Source: CAD feature listing. Evaluate the final solid. Frame: model axes, mm. Face numbers are marked on the shaded views. A direction names the side the tool comes from. Round coordinates to 2 decimals unless told otherwise and drop trailing zeros. Order: outer loops, then holes, each group sorted by start corner. A loop starts at its lowest first (then second) coordinate and runs counter-clockwise, first axis right, second up. Notation, with made-up numbers: (-21, 54) - (19, 54) arc R21 cw to (19, 69) - close; hole circle Ø7 at (15.25, -9.5). An arc over 180 degrees is marked (long way). Return JSON: item names as keys, results as strings. Group by question number.
1) Access query for the marked faces 4 and 5. Directions: +Z, -Z, +X, -X, +Y, -Y. A direction counts if a zero-diameter tool reaches every point of the face in a straight line with its end or side. Return the directions, or none.
2) Section A-A, the plane x = 40.5. Return loops of the section in (y, z).
3) Mould query, pull axis X, two halves, no side actions, for the marked faces 1, 2 and 3. Classes: pulls with the +X half, pulls with the -X half, needs draft (parallel to the pull), parting line crosses it, or undercut.
4) Section D-D, the plane y = -76.5. Return loops of the section in (x, z), plus the area to 3 significant figures.
5) Section B-B, the plane z = 55. Return loops of the section in (x, y), plus the area to 3 significant figures.
6) Contact query for flat-ended pins moving along their axis: P1, Ø1.8, axis at y = -210, z = 65, coming from the +X side; P2, Ø12, axis at x = 167, z = 15, coming from the -Y side; P3, Ø2, axis at x = 236.5, z = 22, coming from the -Y side; P4, Ø1.8, axis at y = -210, z = 56.5, coming from the -X side. Output: stop coordinate, or through.
7) Section C-C, the plane z = 24. Return loops of the section in (x, y), plus the area to 3 significant figures.
8) Ray query, line 1 (X direction, y = -23.5, z = 40); line 2 (Y direction, x = -29, z = 85); line 3 (Z direction, x = 179.5, y = -192.5). Return the intervals inside material, ascending. Write a range as from..to.
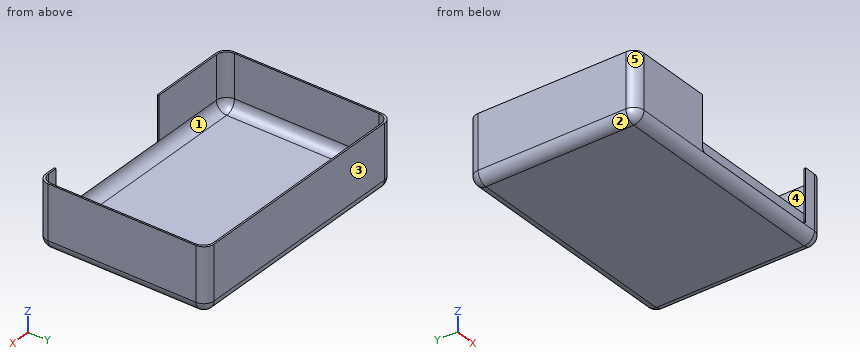
```python
from build123d import *

# Parameters (mm, degrees)
BOSS_EXTRUDE1_DEPTH = 88.9
CUT_EXTRUDE1_DEPTH  = 73.914
FILLET1_R           = 14.224
FILLET2_R           = 14.224
CUT_EXTRUDE2_DEPTH  = 2.286


with BuildPart() as part:
    # Sketch1 → Boss-Extrude1 (new body)
    with BuildSketch(Plane.XY):
        with BuildLine():
            Line((-41.405944168, 22.056216238), (266.696055832, 22.056216238))
            ThreePointArc((266.696055832, 22.056216238), (276.753942688, 17.890103094), (280.920055832, 7.832216238))
            Line((280.920055832, 7.832216238), (280.920055832, -197.145783762))
            ThreePointArc((280.920055832, -197.145783762), (276.753942688, -207.203670617), (266.696055832, -211.369783762))
            Line((266.696055832, -211.369783762), (-41.405944168, -211.369783762))
            ThreePointArc((-41.405944168, -211.369783762), (-51.463831024, -207.203670617), (-55.629944168, -197.145783762))
            Line((-55.629944168, -197.145783762), (-55.629944168, 7.832216238))
            ThreePointArc((-55.629944168, 7.832216238), (-51.463831024, 17.890103094), (-41.405944168, 22.056216238))
        make_face()
    extrude(amount=BOSS_EXTRUDE1_DEPTH)

    # Sketch4 → Cut-Extrude1 (cut)
    with BuildSketch(Plane.XY.offset(88.9)):
        with BuildLine():
            Line((-39.119944168, -209.083783762), (264.410055832, -209.083783762))
            ThreePointArc((264.410055832, -209.083783762), (274.467942688, -204.917670617), (278.634055832, -194.859783762))
            Line((278.634055832, -194.859783762), (278.634055832, 5.546216238))
            ThreePointArc((278.634055832, 5.546216238), (274.467942688, 15.604103094), (264.410055832, 19.770216238))
            Line((264.410055832, 19.770216238), (-39.119944168, 19.770216238))
            ThreePointArc((-39.119944168, 19.770216238), (-49.177831024, 15.604103094), (-53.343944168, 5.546216238))
            Line((-53.343944168, 5.546216238), (-53.343944168, -194.859783762))
            ThreePointArc((-53.343944168, -194.859783762), (-49.177831024, -204.917670617), (-39.119944168, -209.083783762))
        make_face()
    extrude(amount=-CUT_EXTRUDE1_DEPTH, mode=Mode.SUBTRACT)

    # Fillet1
    fillet1_edges = [part.edges().sort_by_distance(p)[0] for p in [
        (-49.177831024, -204.917670617, 14.986),
        (-53.343944168, -94.656783762, 14.986),
        (-49.177831024, 15.604103094, 14.986),
        (112.645055832, 19.770216238, 14.986),
        (274.467942688, 15.604103094, 14.986),
        (278.634055832, -94.656783762, 14.986),
        (274.467942688, -204.917670617, 14.986),
        (112.645055832, -209.083783762, 14.986),
    ]]
    fillet(fillet1_edges, radius=FILLET1_R)

    # Fillet2
    fillet2_edges = [part.edges().sort_by_distance(p)[0] for p in [
        (-55.629944168, -94.656783762, 0),
        (-51.463831024, 17.890103094, 0),
        (112.645055832, 22.056216238, 0),
        (276.753942688, 17.890103094, 0),
        (280.920055832, -94.656783762, 0),
        (276.753942688, -207.203670617, 0),
        (112.645055832, -211.369783762, 0),
        (-51.463831024, -207.203670617, 0),
    ]]
    fillet(fillet2_edges, radius=FILLET2_R)

    # Sketch5 → Cut-Extrude2 (cut)
    with BuildSketch(Plane(origin=(0, -211.369783762, 0), x_dir=(-1, 0, 0), z_dir=(0, -1, 0))):
        with BuildLine():
            Line((-69.838151491, -14.224), (-245.885767903, -14.224))
            ThreePointArc((-245.885767903, -14.224), (-249.477870351, -15.711897552), (-250.965767903, -19.304))
            Line((-250.965767903, -19.304), (-250.965767903, -88.9))
            Line((-250.965767903, -88.9), (-64.758151491, -88.9))
            Line((-64.758151491, -88.9), (-64.758151491, -19.304))
            ThreePointArc((-64.758151491, -19.304), (-66.246049042, -15.711897552), (-69.838151491, -14.224))
        make_face()
    extrude(amount=-CUT_EXTRUDE2_DEPTH, mode=Mode.SUBTRACT)


solid = part.part
```
Geometry check:
{
 "1": {"face 4": "+Z", "face 5": "+Z, -Z, -X, -Y"},
 "2": {"outline": "(-211.37, 14.22) arc R14.22 ccw to (-197.15, 0) - (7.83, 0) arc R14.22 ccw to (22.06, 14.22) - (22.06, 88.9) - (19.77, 88.9) - (19.77, 29.21) arc R14.22 cw to (5.55, 14.99) - (-194.86, 14.99) arc R14.22 cw to (-209.08, 29.21) - (-209.08, 88.9) - (-211.37, 88.9) - close"},
 "3": {"face 1": "undercut", "face 2": "pulls with the -X half", "face 3": "needs draft"},
 "4": {"outline": "(-55.63, 14.22) arc R14.22 ccw to (-41.41, 0) - (266.7, 0) arc R14.22 ccw to (280.92, 14.22) - (280.92, 88.9) - (278.63, 88.9) - (278.63, 29.21) arc R14.22 cw to (264.41, 14.99) - (-39.12, 14.99) arc R14.22 cw to (-53.34, 29.21) - (-53.34, 88.9) - (-55.63, 88.9) - close", "area": "5,380 mm2"},
 "5": {"outline": "(-55.63, -197.15) arc R14.22 ccw to (-41.41, -211.37) - (64.76, -211.37) - (64.76, -209.08) - (-39.12, -209.08) arc R14.22 cw to (-53.34, -194.86) - (-53.34, 5.55) arc R14.22 cw to (-39.12, 19.77) - (264.41, 19.77) arc R14.22 cw to (278.63, 5.55) - (278.63, -194.86) arc R14.22 cw to (264.41, -209.08) - (250.97, -209.08) - (250.97, -211.37) - (266.7, -211.37) arc R14.22 ccw to (280.92, -197.15) - (280.92, 7.83) arc R14.22 ccw to (266.7, 22.06) - (-41.41, 22.06) arc R14.22 ccw to (-55.63, 7.83) - close", "area": "2,160 mm2"},
 "6": {"P1": "x = 274.4", "P2": "y = -211.37", "P3": "y = -209.08", "P4": "x = -49.11"},
 "7": {"outline": "(-55.63, -197.15) arc R14.22 ccw to (-41.41, -211.37) - (64.76, -211.37) - (64.76, -209.08) - (250.97, -209.08) - (250.97, -211.37) - (266.7, -211.37) arc R14.22 ccw to (280.92, -197.15) - (280.92, 7.83) arc R14.22 ccw to (266.7, 22.06) - (-41.41, 22.06) arc R14.22 ccw to (-55.63, 7.83) - close; hole (-52.36, -194.86) arc R13.24 ccw to (-39.12, -208.1) - (264.41, -208.1) arc R13.24 ccw to (277.65, -194.86) - (277.65, 5.55) arc R13.24 ccw to (264.41, 18.78) - (-39.12, 18.78) arc R13.24 ccw to (-52.36, 5.55) - close", "area": "3,240 mm2"},
 "8": {"line 1": "-55.63..-53.34, 278.63..280.92", "line 2": "-211.37..-209.08, 19.77..22.06", "line 3": "0..14.99"}
}
